from build123d import *

# Parameters (mm, degrees)
F0_W     = 12
F0_H     = 5.5
F1_DEPTH = 19.5
F3_R     = 13
F4_DEPTH = 26.45
F5_R     = 4.445
F6_DEPTH = 13.95
F9_DEPTH = 12.55


with BuildPart() as f1:
    # F0 (on Front) → F1 (new body)
    with BuildSketch(Plane.XZ):
        Rectangle(F0_W, F0_H)
    extrude(amount=-F1_DEPTH)

    # F3 (on offset) → F4 (join, through all)
    with BuildSketch(Plane.XZ.offset(6.95)):
        with Locations((0, 9.3)):
            Circle(F3_R)
    extrude(amount=-F4_DEPTH)

    # F5 (on offset) → F6 (join)
    with BuildSketch(Plane.XZ.offset(6.95)):
        with Locations((0, 9.3)):
            Circle(F5_R)
    extrude(amount=F6_DEPTH)

    # F8 (on offset) → F9 (join)
    with BuildSketch(Plane.XZ.offset(20.9)):
        with BuildLine():
            ThreePointArc((0, 4.855), (3.1430896424, 6.1569103576), (4.445, 9.3))
            ThreePointArc((4.445, 9.3), (4.3199432386, 10.3469553071), (3.951809712, 11.335))
            Line((3.951809712, 11.335), (0, 11.335))
            Line((0, 11.335), (0, 4.855))
        make_face()
        with BuildLine():
            ThreePointArc((-3.951809712, 11.335), (-3.7949703556, 6.9856480389), (0, 4.855))
            Line((0, 4.855), (0, 11.335))
            Line((0, 11.335), (-3.951809712, 11.335))
        make_face()
    extrude(amount=F9_DEPTH)


solid = f1.part
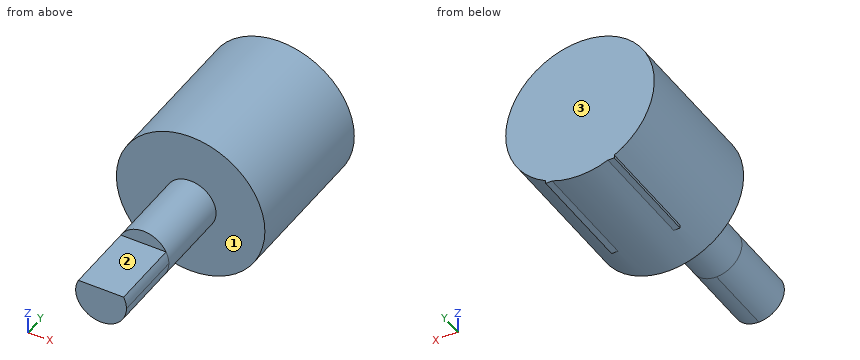
Verification items for the finished model (mm, model axes). Face numbers are marked on the shaded views. A direction names the side the tool comes from. Give positions to 0.01 mm unless a question says otherwise; leave off trailing zeros. Loops run counter-clockwise (first coordinate to the right, second up) from the corner with the lowest first, then second, coordinate; pieces in that order, holes last. Notation, with made-up numbers: (18.5, 80) - (65.5, 80) arc R27 cw to (65.5, 104) - close; hole circle Ø10 at (42.5, 51). An arc over 180 degrees is marked (long way). Write each question's results on one line, items separated by ' | '.
1) Tool access check on the marked faces 1, 2 and 3. Record the directions out of +Z, -Z, +X, -X, +Y, -Y that give a thin tool (end or side, any length) a straight path to the whole face; none if there is none.
Solution:
face 1: -Y | face 2: +Z, +X, -X, -Y | face 3: +Z, -Z, +X, -X, +Y
2) Sectioned sample at C-C on z = 18. Record the boundary of the cut face in (x, y).
Solution:
outline: (-9.66, -6.95) - (9.66, -6.95) - (9.66, 19.5) - (-9.66, 19.5) - close
3) Material ranges on L1, parallel to Y at x = 3, z = 18; L2, parallel to Z at x = 0.25, y = -22 (3 decimals); L3, parallel to Z at x = 0, y = -16 (3 decimals), recorded low to high. Write a range as from..to.
Solution:
L1: -6.95..19.5 | L2: 4.862..11.335 | L3: 4.855..13.745
4) Sectioned sample at A-A on y = 15. Record the boundary of the cut face in (x, z).
Solution:
outline: (-6, -2.75) - (-4.88, -2.75) arc R13 ccw to (4.88, -2.75) - (6, -2.75) - (6, -2.23) arc R13 ccw (long way) to (-6, -2.23) - close
5) Sectioned sample at B-B on x = 8. Record the boundary of the cut face in (y, z).
Solution:
outline: (-6.95, -0.95) - (19.5, -0.95) - (19.5, 19.55) - (-6.95, 19.55) - close
6) Depth check by flat-ended pin: P1, Ø6.5, axis at x = 2, y = -25, coming from the +Z side (3 decimals); P2, Ø5, axis at y = 1, z = 4, coming from the -X side; P3, Ø12, axis at y = -28, z = 4, coming from the -X side (3 decimals). Enter the tip coordinate at first touch or a pass-through.
Solution:
P1: z = 11.335 | P2: x = -12.69 | P3: x = -4.445
